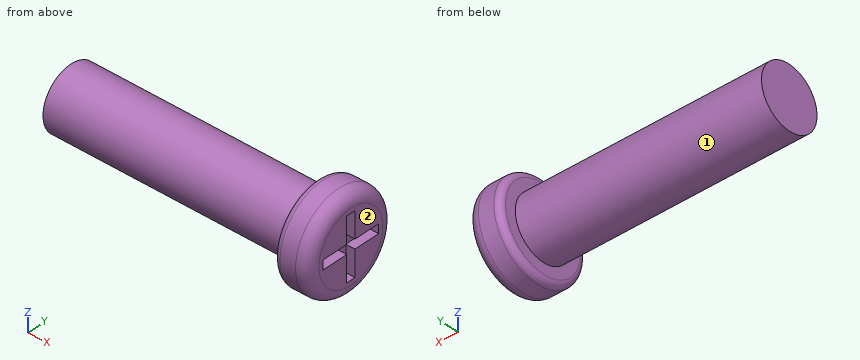
```python
from build123d import *

# Parameters (mm, degrees)
ESBO_O1_R                = 1
RESSALTO_EXTRUS_O1_DEPTH = 25
ESBO_O2_R                = 1.55
RESSALTO_EXTRUS_O2_DEPTH = 1.1
SKETCH1_R                = 1
CUT_EXTRUDE1_DEPTH       = 17
SKETCH2_W                = 0.85
SKETCH2_H                = 0.3
SKETCH2_W_2              = 0.3
SKETCH2_H_2              = 0.85
CUT_EXTRUDE3_DEPTH       = 0.3
FILLET1_R                = 0.4
FILLET2_R                = 0.2


with BuildPart() as part:
    # Esboço1 → Ressalto-extrusão1 (new body)
    with BuildSketch(Plane(origin=(0, 0, 0), x_dir=(0, 0, -1), z_dir=(1, 0, 0))):
        Circle(ESBO_O1_R)
    extrude(amount=RESSALTO_EXTRUS_O1_DEPTH)

    # Esboço2 → Ressalto-extrusão2 (add)
    with BuildSketch(Plane(origin=(25, 0, 0), x_dir=(0, 0, -1), z_dir=(1, 0, 0))):
        Circle(ESBO_O2_R)
    extrude(amount=RESSALTO_EXTRUS_O2_DEPTH)

    # Sketch1 → Cut-Extrude1 (cut)
    with BuildSketch(Plane.ZY):
        Circle(SKETCH1_R)
    extrude(amount=-CUT_EXTRUDE1_DEPTH, mode=Mode.SUBTRACT)

    # Sketch2 → Cut-Extrude3 (cut)
    with BuildSketch(Plane(origin=(26.1, 0, 0), x_dir=(0, 0, -1), z_dir=(1, 0, 0))):
        with Locations((0.575, 0)):
            Rectangle(SKETCH2_W, SKETCH2_H)
        with Locations((-0.575, 0)):
            Rectangle(SKETCH2_W, SKETCH2_H)
        with Locations((0, 0.575)):
            Rectangle(SKETCH2_W_2, SKETCH2_H_2)
        with Locations((0, -0.575)):
            Rectangle(SKETCH2_W_2, SKETCH2_H_2)
        Rectangle(SKETCH2_W_2, SKETCH2_H)
    extrude(amount=-CUT_EXTRUDE3_DEPTH, mode=Mode.SUBTRACT)

    # Fillet1
    fillet1_edges = [part.edges().sort_by_distance(p)[0] for p in [
        (26.1, 0, 1.55),
    ]]
    fillet(fillet1_edges, radius=FILLET1_R)

    # Fillet2
    fillet2_edges = [part.edges().sort_by_distance(p)[0] for p in [
        (25, 0, 1.55),
    ]]
    fillet(fillet2_edges, radius=FILLET2_R)


solid = part.part
```
Verification items for the finished model (mm, model axes). Face numbers are marked on the shaded views. A direction names the side the tool comes from. Round coordinates to 2 decimals unless told otherwise and drop trailing zeros. Order: outer loops, then holes, each group sorted by start corner. A loop starts at its lowest first (then second) coordinate and runs counter-clockwise, first axis right, second up.
1) Cross-section at A-A, the plane z = 0. Record the cut outline in (x, y), plus the area to 3 significant figures.
Geometry says:
outline: (17, -1) - (25, -1) - (25, -1.35) arc R0.2 ccw to (25.2, -1.55) - (25.7, -1.55) arc R0.4 ccw to (26.1, -1.15) - (26.1, -1) - (25.8, -1) - (25.8, 1) - (26.1, 1) - (26.1, 1.15) arc R0.4 ccw to (25.7, 1.55) - (25.2, 1.55) arc R0.2 ccw to (25, 1.35) - (25, 1) - (17, 1) - close
area: 18.7 mm2
2) Material ranges on line 1 (Y direction, x = 23.5, z = 0.05); line 2 (X direction, y = -1, z = -0.35); line 3 (X direction, y = 0.1, z = -0.55), recorded low to high.
Geometry says:
line 1: y = -1 to 1
line 2: x = 25 to 26.1
line 3: x = 17 to 25.8
3) Depth check by flat-ended pin: pin 1 (1 mm diameter, centred on x = 22.5, z = 0.5, fed in from -Y); pin 2 (1 mm diameter, centred on x = 19.5, y = 1, fed in from -Z). Enter the tip coordinate at first touch or a pass-through.
Geometry says:
pin 1: stops at y = -1
pin 2: stops at z = -0.87
4) Cross-section at C-C, the plane x = 18.5. Record the cut outline in (y, z).
Geometry says:
outline: circle Ø2 at (0, 0)
5) Tool access check on the marked faces 1 and 2. Record the directions out of +Z, -Z, +X, -X, +Y, -Y that give a thin tool (end or side, any length) a straight path to the whole face; none if there is none.
Geometry says:
face 1: -X
face 2: +Z, -Z, +X, +Y, -Y
